The model under review builds one solid part; all positions refer to its coordinate system, in mm. A direction names the side the tool comes from. Coordinates: 2 decimals unless noted, no trailing zeros. Order: outer loops, then holes, each group sorted by start corner. A loop starts at its lowest first (then second) coordinate and runs counter-clockwise, first axis right, second up. Notation, with made-up numbers: (76.5, -8) - (106.5, -8) arc R20 cw to (106.5, 19) - close; hole circle Ø4 at (-11, 68.5). An arc over 180 degrees is marked (long way). Answer in a Markdown table with one row per item.
Autodesk Fusion 360 part; units mm, degrees
sketch "Sketch1" plane through (0, 0, 0) normal (0, 1, 0) x (1, 0, 0)
  circle A0 centre (0, 0) radius 6
  dimension "d1" = 12
extrude "Extrude1" add sketch "Sketch1" along normal blind 45
sketch "Sketch2" plane through (0, 0, 0) normal (0, -1, 0) x (1, 0, 0)
  circle A0 centre (0, 0) radius 6
  circle A1 centre (0, 0) radius 1.6031
  circle A2 centre (0, 0) radius 2.5
  circle A3 centre (0, 0) radius 2
  dimension "d4" = 5
  dimension "d5" = 4
extrude "Extrude2" cut sketch "Sketch2" against normal blind 5.5 contours A2
extrude "Extrude3" cut 1 faces at (1.1392, 0, 0.5006) along direction (0, 1, 0) blind 71
sketch "Sketch3" plane through (0, 45, 0) normal (0, 1, 0) x (-1, 0, 0)
  circle A0 centre (0, 0) radius 2
  circle A1 centre (0, 0) radius 6
  circle A2 centre (0, 0) radius 2.75
  dimension "d10" = 5.5
extrude "Extrude4" cut sketch "Sketch3" against normal blind 24 contours A2
ref_plane "WorkPlane1" through (0, 39, 0) normal (0, 1, 0) x (1, 0, 0)
sketch "Sketch4" plane through (0, 39, 0) normal (0, 1, 0) x (1, 0, 0)
  line L0 (4, 2.3094) -> (0, 4.6188)
  line L1 (0, 4.6188) -> (-4, 2.3094)
  line L2 (-4, 2.3094) -> (-4, -2.3094)
  line L3 (-4, -2.3094) -> (0, -4.6188)
  line L4 (0, -4.6188) -> (4, -2.3094)
  line L5 (4, -2.3094) -> (4, 2.3094)
  line L6 (4, -2.3094) -> (4, -7)
  line L7 (4, -7) -> (-4.1244, -7)
  line L8 (-4.1244, -7) -> (-4, -2.3094)
  dimension "d14" = 4
extrude "Extrude5" cut sketch "Sketch4" against normal blind 4.2
Item 1: Mouldability with a two-part tool opening along Y and no side actions: class faces 4 (the face through (2.028, 36.929, -3.448)), 5 (the face through (-1, 21, -2)), 6 (the face through (0, 34.8, 3)), 7 (the face through (3, 0, 0)) as +Y half, -Y half, draft (parallel to the pull), parting line (faces both ways), or undercut.
Check values:
| item | result |
|---|---|
| face 4 | undercut |
| face 5 | +Y half |
| face 6 | undercut |
| face 7 | -Y half |
Item 2: To check wall thickness, follow line 1 (Z direction, x = 0, y = 3.15); line 2 (Y direction, x = -1.25, z = -1.75); line 3 (Y direction, x = -0.25, z = 4.25). State the ranges of each line that lie inside material, in increasing order. Write a range as from..to.
Check values:
| item | result |
|---|---|
| line 1 | -6..-2.5, 2.5..6 |
| line 2 | 5.5..21 |
| line 3 | 0..34.8, 39..45 |
Item 3: We need section A-A, the plane z = 0. Write out the cut boundary in (x, y), then the cut area to 3 significant figures.
Check values:
| item | result |
|---|---|
| outline | (-6, 0) - (-2.5, 0) - (-2.5, 5.5) - (-2, 5.5) - (-2, 21) - (-2.75, 21) - (-2.75, 34.8) - (-4, 34.8) - (-4, 39) - (-2.75, 39) - (-2.75, 45) - (-6, 45) - close; (2, 5.5) - (2.5, 5.5) - (2.5, 0) - (6, 0) - (6, 45) - (2.75, 45) - (2.75, 39) - (4, 39) - (4, 34.8) - (2.75, 34.8) - (2.75, 21) - (2, 21) - close |
| area | 308 mm^2 |
Item 4: We need section B-B, the plane y = 19. Write out the cut boundary in (x, z), then the cut area to 3 significant figures.
Check values:
| item | result |
|---|---|
| outline | circle Ø12 at (0, 0); hole circle Ø4 at (0, 0) |
| area | 101 mm^2 |
Item 5: Tool access review of faces 1 (the face through (4, 37, 1)), 2 (the face through (-1, 5.5, 2)), 3 (the face through (0.596, 42.042, -2.685)): name each direction out of +Z, -Z, +X, -X, +Y, -Y from which nothing blocks a thin tool from reaching the whole face with its end or side.
Check values:
| item | result |
|---|---|
| face 1 | +Z |
| face 2 | -Y |
| face 3 | +Y |
Item 6: We need section D-D, the plane z = -3.5. Write out the cut boundary in (x, y), then the cut area to 3 significant figures.
Check values:
| item | result |
|---|---|
| outline | (-4.87, 0) - (4.87, 0) - (4.87, 45) - (-4.87, 45) - close; hole (-1.94, 34.8) - (1.94, 34.8) - (1.94, 39) - (-1.94, 39) - close |
| area | 422 mm^2 |
Item 7: We need section C-C, the plane x = -3.5. Write out the cut boundary in (y, z), then the cut area to 3 significant figures.
Check values:
| item | result |
|---|---|
| outline | (0, -4.87) - (45, -4.87) - (45, 4.87) - (39, 4.87) - (39, -2.6) - (34.8, -2.6) - (34.8, 4.87) - (0, 4.87) - close |
| area | 407 mm^2 |
Item 8: Clearance check with flat-ended pins moving along their axes: pin 1 Ø4.5 at (x, z) = (0, 0) entering from -Y; pin 2 Ø1.5 at (x, y) = (-4, 28) entering from -Z; pin 3 Ø2 at (y, z) = (36.5, 1.5) entering from -X. State where each tip first meets the part, or that it passes through.
Check values:
| item | result |
|---|---|
| pin 1 | y = 5.5 |
| pin 2 | z = -5.04 |
| pin 3 | x = -5.98 |
